For this review, take the finished solid that the model builds, in its own axes (mm). A direction names the side the tool comes from. Give positions to 0.01 mm unless a question says otherwise; leave off trailing zeros. Write each loop counter-clockwise with the first axis right and the second up, starting at its lowest first coordinate (ties: lowest second). Pieces come first, ordered by that corner, then holes. Notation, with made-up numbers: M 79.5,5.5 L 84.5,5.5 A33 cw 84.5,37.5 Z; hole C 27,79.5 d9. An arc over 180 degrees is marked long. One line per item, written item: value. Start each with the question number.
Item 1: Mouldability with a two-part tool opening along X and no side actions: class faces 4 (the face through (-3.21, 6.56, 0.32)), 5 (the face through (0, 3, 0)), 6 (the face through (1.88, 7.46, 5.96)), 7 (the face through (-4.2, -1.9, -2)) as released by +X, released by -X, zero draft, split by the parting line, or undercut.
Item 2: Consider section D-D, the plane y = 2.75. Write out the cut boundary in (x, z).
Item 3: To check wall thickness, follow probe 1 along X at (y, z) = (-1.2, 0); probe 2 along Z at (x, y) = (4.75, -0.5); probe 3 along X at (y, z) = (5.75, -5.25). State the ranges of each line that lie inside material, in increasing order.
Item 4: Clearance check with flat-ended pins moving along their axes: pin 1 Ø6 at (x, z) = (0, 0) entering from -Y; pin 2 Ø4 at (x, z) = (-5.78, 5.53) entering from +Y; pin 3 Ø2 at (x, y) = (-0.5, 8) entering from -Z; pin 4 Ø0.6 at (y, z) = (3, 0) entering from -X. State where each tip first meets the part, or that it passes through.
Item 5: Consider section C-C, the plane x = 6.5. Give the number of separate pieces and of enclosed holes in the cut face, and give its area (3 significant figures).
Item 6: Tool access review of faces 1 (the face through (0, 0, 0)), 2 (the face through (0, 10.5, 3)), 3 (the face through (-3, 2.5, 0)): name each direction out of +Z, -Z, +X, -X, +Y, -Y from which nothing blocks a thin tool from reaching the whole face with its end or side.
Item 7: Consider section A-A, the plane y = 1. Write out the cut boundary in (x, z), and give its area (3 significant figures).
Item 8: Consider section B-B, the plane y = 6.5. Write out the cut boundary in (x, z), and give its area (3 significant figures).
```python
from build123d import *

# Parameters (mm, degrees)
SKETCH1_R               = 9.75
SKETCH1_R_2             = 1.25
BOSS_EXTRUDE2_DEPTH     = 2
SKETCH2_R               = 6.25
BOSS_EXTRUDE3_DEPTH     = 8.5
SKETCH4_R               = 2.5
CUT_EXTRUDE1_DEPTH      = 7.5
CUT_EXTRUDE2_DEPTH      = 7.5
CUT_EXTRUDE2_DEPTH_BACK = 6.75
SKETCH5_R               = 1.75
BOSS_EXTRUDE5_START     = 1.9
SKETCH7_R               = 9.75
SKETCH7_R_2             = 4.5
SKETCH7_R_3             = 1.25
BOSS_EXTRUDE5_DEPTH     = 1.9
CUT_EXTRUDE3_DEPTH      = 8
FILLET1_R               = 2.5


with BuildPart() as part:
    # Sketch1 → Boss-Extrude2 (new body)
    with BuildSketch(Plane(origin=(0, 0, 0), x_dir=(1, 0, 0), z_dir=(0, 1, 0))):
        with Locations(Location((0, 0, 0), (0, 0, 270))):
            Circle(SKETCH1_R)
        with Locations(Location((-5.78230038, 5.52856241, 0), (0, 0, 270))):
            Circle(SKETCH1_R_2, mode=Mode.SUBTRACT)
        with Locations(Location((-5.78230038, -5.52856241, 0), (0, 0, 270))):
            Circle(SKETCH1_R_2, mode=Mode.SUBTRACT)
        with Locations(Location((5.78230038, -5.52856241, 0), (0, 0, 270))):
            Circle(SKETCH1_R_2, mode=Mode.SUBTRACT)
        with Locations(Location((5.78230038, 5.52856241, 0), (0, 0, 270))):
            Circle(SKETCH1_R_2, mode=Mode.SUBTRACT)
    extrude(amount=BOSS_EXTRUDE2_DEPTH)

    # Sketch2 → Boss-Extrude3 (add)
    with BuildSketch(Plane(origin=(0, 2, 0), x_dir=(1, 0, 0), z_dir=(0, 1, 0))):
        with Locations(Location((0, 0, 0), (0, 0, 270))):
            Circle(SKETCH2_R)
    extrude(amount=BOSS_EXTRUDE3_DEPTH)

    # Sketch4 → Cut-Extrude1 (cut)
    with BuildSketch(Plane(origin=(0, 10.5, 0), x_dir=(1, 0, 0), z_dir=(0, 1, 0))):
        with Locations(Location((0, 0, 0), (0, 0, 270))):
            Circle(SKETCH4_R)
    extrude(amount=-CUT_EXTRUDE1_DEPTH, mode=Mode.SUBTRACT)

    # Sketch5 → Cut-Extrude2 (cut, two sides: drawn at the far end of the back side and taken through both)
    with BuildSketch(Plane.XY.offset(-CUT_EXTRUDE2_DEPTH_BACK)):
        with Locations(Location((0, 6.914506731, 0), (0, 0, 180))):
            Circle(SKETCH5_R)
    extrude(amount=CUT_EXTRUDE2_DEPTH + CUT_EXTRUDE2_DEPTH_BACK, mode=Mode.SUBTRACT)

    # Sketch7 → Boss-Extrude5 (add)
    with BuildSketch(Plane.XZ.offset(BOSS_EXTRUDE5_START)):
        with Locations(Location((0, 0, 0), (0, 0, 270))):
            Circle(SKETCH7_R)
        with Locations(Location((0, 0, 0), (0, 0, 90))):
            Circle(SKETCH7_R_2, mode=Mode.SUBTRACT)
        with Locations(Location((-5.78230038, 5.52856241, 0), (0, 0, 270))):
            Circle(SKETCH7_R_3, mode=Mode.SUBTRACT)
        with Locations(Location((5.78230038, 5.52856241, 0), (0, 0, 270))):
            Circle(SKETCH7_R_3, mode=Mode.SUBTRACT)
        with Locations(Location((5.78230038, -5.52856241, 0), (0, 0, 270))):
            Circle(SKETCH7_R_3, mode=Mode.SUBTRACT)
        with Locations(Location((-5.78230038, -5.52856241, 0), (0, 0, 270))):
            Circle(SKETCH7_R_3, mode=Mode.SUBTRACT)
    extrude(amount=-BOSS_EXTRUDE5_DEPTH)

    # Sketch9 → Cut-Extrude3 (cut)
    with BuildSketch(Plane(origin=(0, 10.5, 0), x_dir=(1, 0, 0), z_dir=(0, 1, 0))):
        Polygon((-2.414753661, -0.64727487), (-2.414753661, 0.64727487), (-3.984419716, 0), align=None)
    extrude(amount=-CUT_EXTRUDE3_DEPTH, mode=Mode.SUBTRACT)

    # Fillet1
    # the kernel refuses this fillet: 2.5 mm, written as the material it adds along each edge
    with BuildSketch(Plane(origin=(0, 2, 0), x_dir=(0, 0, 1), z_dir=(-1, 0, 0))) as fillet1_piece_1_section:
        with BuildLine():
            CenterArc((6.25 + FILLET1_R, FILLET1_R), FILLET1_R, 180, 90)
            Line((6.25, FILLET1_R), (6.25, 0))
            Line((6.25, 0), (6.25 + FILLET1_R, 0))
        make_face()
    fillet1_piece_1 = revolve(axis=Axis((0, 2, 0), (0, 1, 0)), mode=Mode.PRIVATE)
    fillet1_piece_1 = fillet1_piece_1 - Plane(origin=(-5.78230038, 2.704024644, 5.52856241), x_dir=(0, 0, 1), z_dir=(0, -1, 0)) * Cylinder(1.25, 35, mode=Mode.PRIVATE)
    fillet1_piece_1 = fillet1_piece_1 - Plane(origin=(5.78230038, 2.704024644, 5.52856241), x_dir=(0, 0, 1), z_dir=(0, -1, 0)) * Cylinder(1.25, 35, mode=Mode.PRIVATE)
    fillet1_piece_1 = fillet1_piece_1 - Plane(origin=(-5.78230038, 2.704024644, -5.52856241), x_dir=(0, 0, 1), z_dir=(0, -1, 0)) * Cylinder(1.25, 35, mode=Mode.PRIVATE)
    fillet1_piece_1 = fillet1_piece_1 - Plane(origin=(5.78230038, 2.704024644, -5.52856241), x_dir=(0, 0, 1), z_dir=(0, -1, 0)) * Cylinder(1.25, 35, mode=Mode.PRIVATE)
    add(fillet1_piece_1)


solid = part.part
```
Model answer:
1. face 4: undercut
1. face 5: undercut
1. face 6: split by the parting line
1. face 7: zero draft
2. outline: M -5.46,-4.32 A1.25 cw -4.56,-5.26 A6.96 ccw 4.56,-5.26 A1.25 cw 5.46,-4.32 A6.96 ccw 5.46,4.32 A1.25 cw 4.56,5.26 A6.96 ccw -4.56,5.26 A1.25 cw -5.46,4.32 A6.96 ccw Z; hole M -3.98,0 L -2.41,-0.65 L -2.41,0.65 Z
3. probe 1: x = -9.75 to -4.5, 4.5 to 9.75
3. probe 2: z = -8.51 to -6.23, -4.82 to 4.82, 6.23 to 8.51
3. probe 3: x = -3.39 to -1.31, 1.31 to 3.39
4. pin 1: stops at y = 0
4. pin 2: stops at y = 10.5
4. pin 3: stops at z = -6.25
4. pin 4: stops at x = -7.02
5. separate pieces: 3
5. enclosed holes: 0
5. area: 48.2 mm2
6. face 1: -Y
6. face 2: +Z, -Z, +X, -X, +Y
6. face 3: +Y
7. outline: C 0,0 d19.5; hole C -5.78,-5.53 d2.5; hole C -5.78,5.53 d2.5; hole C 5.78,-5.53 d2.5; hole C 5.78,5.53 d2.5
7. area: 279 mm2
8. outline: M -3.98,0 L -2.41,0.65 A2.5 cw -1.7,1.83 L -1.7,6.01 A6.25 ccw -1.7,-6.01 L -1.7,-1.83 A2.5 cw -2.41,-0.65 Z; M 1.7,-6.01 A6.25 ccw 1.7,6.01 L 1.7,1.83 A2.5 cw 1.7,-1.83 Z
8. area: 75.7 mm2
